Verification items for the finished model (mm, model axes). Give positions to 0.01 mm unless a question says otherwise; leave off trailing zeros. Order: outer loops, then holes, each group sorted by start corner. A loop starts at its lowest first (then second) coordinate and runs counter-clockwise, first axis right, second up. Notation, with made-up numbers: (34.25, 30.25) -> (85.25, 30.25) arc R6 cw to (85.25, 38.25) -> close; hole circle Ø1 at (77.25, 58.5). An arc over 180 degrees is marked (long way). One line per question, with ' | ' between items. Start each with the question number.
Q1. Section check C-C on x = 24. Record the cut outline in (y, z), plus the area to 3 significant figures.
Q2. Go/stop test with flat-tipped pins: pin 1 (1 mm diameter, centred on y = 2, z = -32, fed in from -X); pin 2 (3 mm diameter, centred on x = -31.2, z = -16.63, fed in from -Y). Record where each tip stops, or that it passes through.
Q3. Section check B-B on y = 2.3. Give the number of separate pieces and of enclosed holes in the cut face, plus the area to 3 significant figures.
Q4. Section check D-D on z = 37. Record the cut outline in (x, y).
Q5. Section check A-A on z = 15.5. Record the cut outline in (x, y), plus the area to 3 significant figures.
Q6. Material ranges on probe 1 along Z at (x, y) = (-15.5, 0.9); probe 2 along Z at (x, y) = (-35, 2.75); probe 3 along Z at (x, y) = (-50, 1.8), recorded low to high. Write a range as [from, to].
from build123d import *

# Parameters (mm, degrees)
SKETCH_10_R         = 2.35
EXTRUDE_2_DEPTH     = 3
CUT_EXTRUDE_3_DEPTH = 3


with BuildPart() as part:
    # 草图10 → 凸台-拉伸2 (new body)
    with BuildSketch(Plane(origin=(0, 0, 0), x_dir=(1, 0, 0), z_dir=(0, 1, 0))):
        with BuildLine():
            Line((33.405753886, -43.6927409), (49.102625926, -49.386437869))
            ThreePointArc((49.102625926, -49.386437869), (50.631828553, -49.317990247), (51.664738322, -48.188280923))
            Line((51.664738322, -48.188280923), (70.544015322, 3.859728807))
            ThreePointArc((70.544015322, 3.859728807), (70.4755677, 5.388931433), (69.345858375, 6.421841203))
            Line((69.345858375, 6.421841203), (53.648986335, 12.115538173))
            ThreePointArc((53.648986335, 12.115538173), (18.754387434, 51.703703465), (-33.405753886, 43.6927409))
            Line((-33.405753886, 43.6927409), (-49.102625926, 49.386437869))
            ThreePointArc((-49.102625926, 49.386437869), (-50.631828553, 49.317990247), (-51.664738322, 48.188280923))
            Line((-51.664738322, 48.188280923), (-70.544015322, -3.859728807))
            ThreePointArc((-70.544015322, -3.859728807), (-70.4755677, -5.388931433), (-69.345858375, -6.421841203))
            Line((-69.345858375, -6.421841203), (-53.648986335, -12.115538173))
            ThreePointArc((-53.648986335, -12.115538173), (-18.754387434, -51.703703465), (33.405753886, -43.6927409))
        make_face()
        with Locations(Location((16.22853422, 44.109349089, 0), (0, 0, 270))):
            Circle(SKETCH_10_R, mode=Mode.SUBTRACT)
        with Locations(Location((-44.109349089, 16.22853422, 0), (0, 0, 270))):
            Circle(SKETCH_10_R, mode=Mode.SUBTRACT)
        with Locations(Location((-16.22853422, -44.109349089, 0), (0, 0, 270))):
            Circle(SKETCH_10_R, mode=Mode.SUBTRACT)
        with Locations(Location((44.109349089, -16.22853422, 0), (0, 0, 270))):
            Circle(SKETCH_10_R, mode=Mode.SUBTRACT)
    extrude(amount=EXTRUDE_2_DEPTH)

    # 草图11 → 切除-拉伸3 (cut)
    with BuildSketch(Plane(origin=(0, 0, 0), x_dir=(1, 0, 0), z_dir=(0, 1, 0))):
        with BuildLine():
            Line((14.302948542, -11.889729308), (13.381558854, -11.555515354))
            ThreePointArc((13.381558854, -11.555515354), (11.104938847, -11.342582915), (10.515931052, -9.13319189))
            ThreePointArc((10.515931052, -9.13319189), (12.384418559, -7.81520353), (14.268129897, -9.111340281))
            Line((14.268129897, -9.111340281), (15.189519584, -9.445554235))
            Line((15.189519584, -9.445554235), (14.302948542, -11.889729308))
        make_face()
        with BuildLine():
            Line((17.678018521, 0.289333077), (18.599408209, -0.044880878))
            Line((18.599408209, -0.044880878), (17.712837166, -2.48905595))
            Line((17.712837166, -2.48905595), (16.791447479, -2.154841996))
            ThreePointArc((16.791447479, -2.154841996), (14.514827471, -1.941909558), (13.925819677, 0.267481467))
            ThreePointArc((13.925819677, 0.267481467), (15.794307183, 1.585469828), (17.678018521, 0.289333077))
        make_face()
        with BuildLine():
            Line((-33.104295256, 18.709506556), (-32.182905569, 18.375292602))
            ThreePointArc((-32.182905569, 18.375292602), (-29.317277767, 15.952969139), (-33.069476611, 15.931117529))
            Line((-33.069476611, 15.931117529), (-33.990866299, 16.265331483))
            Line((-33.990866299, 16.265331483), (-33.104295256, 18.709506556))
        make_face()
        with BuildLine():
            Line((-36.514183881, 9.308833199), (-35.592794193, 8.974619245))
            ThreePointArc((-35.592794193, 8.974619245), (-32.727166391, 6.552295782), (-36.479365236, 6.530444172))
            Line((-36.479365236, 6.530444172), (-37.400754923, 6.864658126))
            Line((-37.400754923, 6.864658126), (-36.514183881, 9.308833199))
        make_face()
        Polygon((-24.792131447, 19.63033923), (-31.611908696, 0.828992516), (5.990784733, -12.810561982), (12.810561982, 5.990784733), align=None)
    extrude(amount=CUT_EXTRUDE_3_DEPTH, mode=Mode.SUBTRACT)


solid = part.part
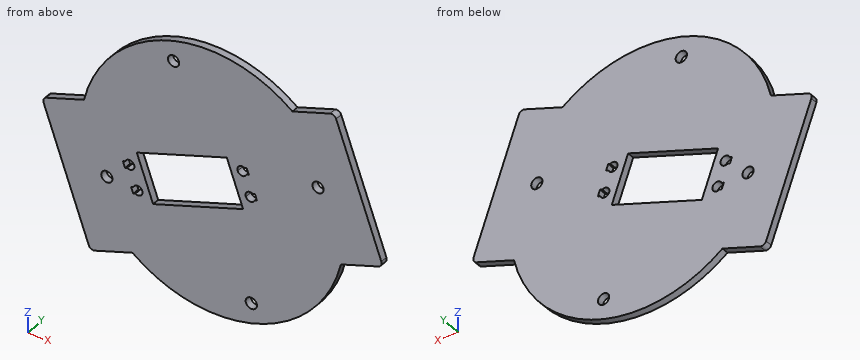
Filled in:
1) outline: (0, -49.49) -> (3, -49.49) -> (3, 49.49) -> (0, 49.49) -> close | area: 297 mm²
2) pin 1: x = -57.72 | pin 2: through
3) separate pieces: 1 | enclosed holes: 9 | area: 10,100 mm²
4) outline: (-40.69, 0) -> (55.72, 0) -> (55.72, 3) -> (-40.69, 3) -> close
5) outline: (-52.77, 0) -> (41.88, 0) -> (41.88, 3) -> (-52.77, 3) -> close; (46.34, 0) -> (63.52, 0) -> (63.52, 3) -> (46.34, 3) -> close | area: 335 mm²
6) probe 1: [-52.77, -16.26], [5.02, 41.88], [46.34, 52.77] | probe 2: [-44.27, -9.2], [-5.27, 42.43] | probe 3: [-49.49, 22.91]
